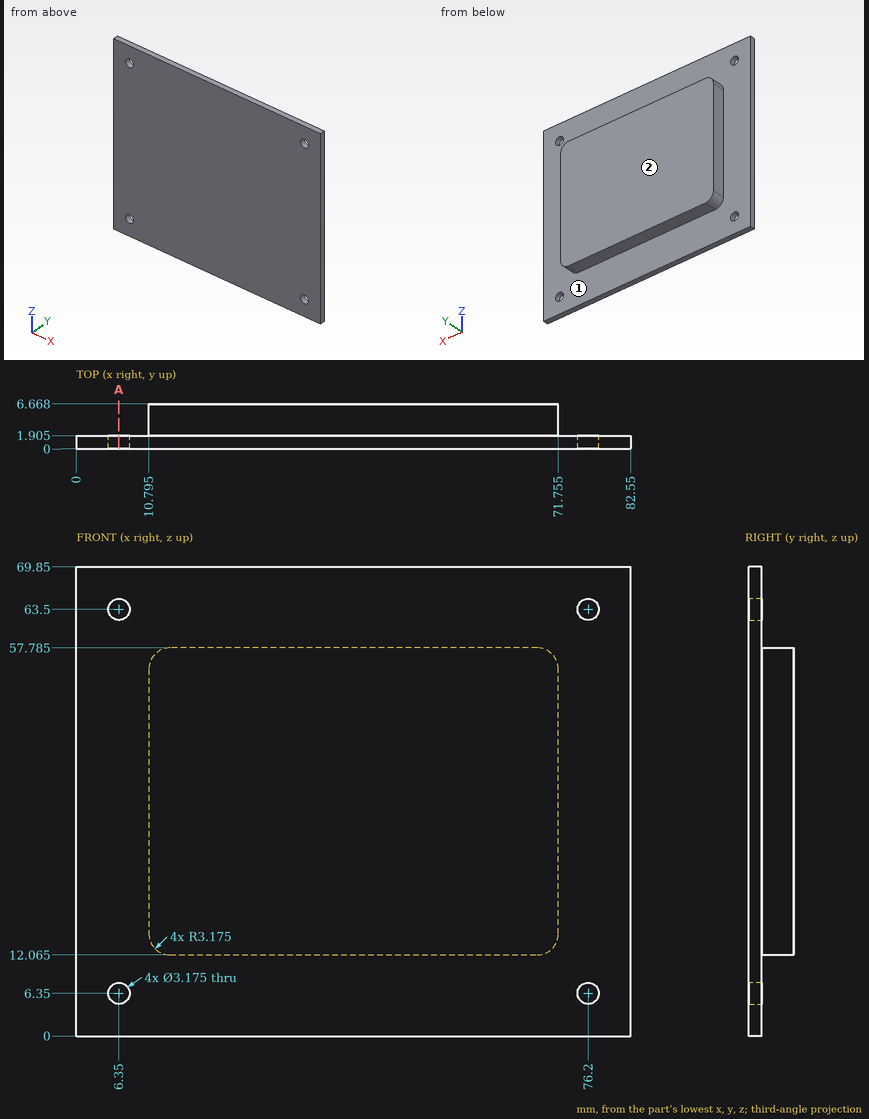
Study the drawing (mm; zero at the part's minimum x, y, z) and answer. A direction names the side the tool comes from. Give positions to 0.01 mm unless a question says otherwise; leave off trailing zeros. Return JSON: item names as keys, results as strings. Group by question number.
1. Find section A-A (x = 6.35). State how many separate pieces and enclosed holes the cut face has, then the cut area to 3 significant figures.
2. Which of the six approach directions +Z, -Z, +X, -X, +Y, -Y give full straight-line access (tool end or side, diameter ignored) to the marked faces 1 and 2?
3. Given pin 1 Ø2.5 at (y, z) = (5.5, 31.5) entering from +X (1 decimal); pin 2 Ø5 at (x, z) = (32, 20) entering from -Y; pin 3 Ø1.4 at (y, z) = (4, 38.5) entering from -X (1 decimal); pin 4 Ø4 at (y, z) = (5, 57) entering from +X, each flat-ended and moving along its own axis, determine where each tip first touches the part or whether it passes through.
4. Straight lines are drawn through the part: line 1 (X direction, y = 1.35, z = 6.35); line 2 (Z direction, x = 76.2, y = 1.3); line 3 (X direction, y = 5.5, z = 25.5) (1 decimal). For each, find the intervals that lie inside material, in ascending order. Write a range as [from, to].
Verdict:
{
 "1": {"separate pieces": "3", "enclosed holes": "0", "area": "121 mm^2"},
 "2": {"face 1": "+Y", "face 2": "+Z, -Z, +X, -X, +Y"},
 "3": {"pin 1": "stops at x = 71.8", "pin 2": "stops at y = 0", "pin 3": "stops at x = 10.8", "pin 4": "stops at x = 71.73"},
 "4": {"line 1": "x = [0, 4.76], [7.94, 74.61], [77.79, 82.55]", "line 2": "z = [0, 4.76], [7.94, 61.91], [65.09, 69.85]", "line 3": "x = [10.8, 71.8]"}
}
